Build history of the part. All positions in model axes, mm. A direction names the side the tool comes from. Round coordinates to 2 decimals unless told otherwise and drop trailing zeros. Order: outer loops, then holes, each group sorted by start corner. A loop starts at its lowest first (then second) coordinate and runs counter-clockwise, first axis right, second up. Notation, with made-up numbers: (51.25, 26) -> (63.25, 26) arc R17 ccw to (63.25, 50) -> close; hole circle Ø5 at (-33.5, 16). An arc over 180 degrees is marked (long way). Answer as a JSON object with one key per item and string values.
from build123d import *

# Parameters (mm, degrees)
SKETCH1_R                = 18
SKETCH1_R_2              = 17.75
BOSS_EXTRUDE1_DEPTH      = 210
BOSS_EXTRUDE2_DEPTH      = 22.5
CUT_EXTRUDE2_DEPTH       = 213.245370912
CUT_EXTRUDE12_START      = -27
CUT_EXTRUDE12_DEPTH      = 23.323952
CUT_EXTRUDE13_REACH      = 217.691
CUT_EXTRUDE13_END_RADIUS = 19.770854308
BOSS_EXTRUDE3_REACH      = 235.245
BOSS_EXTRUDE3_END_RADIUS = 18
BOSS_EXTRUDE3_START      = 21


with BuildPart() as part:
    # Sketch1 → Boss-Extrude1 (new body)
    with BuildSketch(Plane(origin=(0, 0, 0), x_dir=(0, 0, -1), z_dir=(1, 0, 0))):
        Circle(SKETCH1_R)
        Circle(SKETCH1_R_2, mode=Mode.SUBTRACT)
    extrude(amount=BOSS_EXTRUDE1_DEPTH)


with BuildPart() as body_2:
    # Sketch4 → Boss-Extrude2 (new, symmetric)
    with BuildSketch(Plane.ZY.offset(-67)):
        with BuildLine():
            ThreePointArc((-13.779943134, 14.177441493), (7.695629669, 18.21164364), (19.770854308, 0))
            add(Edge.make_bspline(
                [(-13.779943134, 14.177441493), (-10.685751008, 18.612681967), (-3.179720318, 24.881089629), (14.245409909, 21.177624873), (20.93871501, 8.550633365), (19.770854308, 0)],
                knots=[0, 0, 0, 0, 0.331280275, 0.485623577, 1, 1, 1, 1], degree=3))
        make_face()
    extrude(amount=BOSS_EXTRUDE2_DEPTH, both=True)


with BuildPart() as cut_extrude2_tool:
    # Sketch2 → Cut-Extrude2 (new, through all)
    with BuildSketch(Plane(origin=(0, 0, 0), x_dir=(1, 0, 0), z_dir=(0, 1, 0))):
        with BuildLine():
            Line((63, -5), (71, -5))
            ThreePointArc((71, -5), (76, 0), (71, 5))
            Line((71, 5), (63, 5))
            ThreePointArc((63, 5), (58, 0), (63, -5))
        make_face()
    extrude(amount=CUT_EXTRUDE2_DEPTH)


with BuildPart() as part_1:
    add(part.part)

    # Cut-Extrude2: cut by cut_extrude2_tool
    add(cut_extrude2_tool.part, mode=Mode.SUBTRACT)



with BuildPart() as body_2_1:
    add(body_2.part)

    # Cut-Extrude2: cut by cut_extrude2_tool
    add(cut_extrude2_tool.part, mode=Mode.SUBTRACT)

    # Sketch7 → Cut-Extrude12 (cut)
    with BuildSketch(Plane(origin=(0, 27, 0), x_dir=(1, 0, 0), z_dir=(0, 1, 0)).offset(CUT_EXTRUDE12_START)):
        with BuildLine():
            ThreePointArc((46.185450517, -14.355615707), (44.923728597, -8.827176662), (44.5, -3.172441075))
            Line((44.5, -3.172441075), (44.5, -19.93558029))
            Line((44.5, -19.93558029), (67, -19.93558029))
            ThreePointArc((67, -19.93558029), (56.225243913, -18.516387819), (46.185450517, -14.355615707))
        make_face()
        with BuildLine():
            ThreePointArc((87.814549483, -14.355615707), (77.774756087, -18.516387819), (67, -19.93558029))
            Line((67, -19.93558029), (89.5, -19.93558029))
            Line((89.5, -19.93558029), (89.5, -3.172440538))
            ThreePointArc((89.5, -3.172440538), (89.076271443, -8.827176396), (87.814549483, -14.355615707))
        make_face()
    extrude(amount=CUT_EXTRUDE12_DEPTH, mode=Mode.SUBTRACT)

    # Cut-Extrude13: up to this cylinder (the profile starts outside it)
    cut_extrude13_end = Plane(origin=(67, 0, 0), z_dir=(1, 0, 0)) * Cylinder(CUT_EXTRUDE13_END_RADIUS, 512.063876616, mode=Mode.PRIVATE)
    # Sketch7<4> → Cut-Extrude13 (cut, up to the surface)
    with BuildSketch(Plane(origin=(0, 27, 0), x_dir=(1, 0, 0), z_dir=(0, 1, 0)), mode=Mode.PRIVATE) as cut_extrude13_sk1:
        with BuildLine():
            Line((62.018448737, 13.779943134), (44.5, 13.779943134))
            Line((44.5, 13.779943134), (44.5, -3.172441075))
            ThreePointArc((44.5, -3.172441075), (44.781644245, 1.442087549), (45.622395888, 5.98811159))
            ThreePointArc((45.622395888, 5.98811159), (53.132553103, 11.331484209), (62.018448737, 13.779943134))
        make_face()
    cut_extrude13_tool1 = extrude(cut_extrude13_sk1.sketch, amount=-CUT_EXTRUDE13_REACH, mode=Mode.PRIVATE) - cut_extrude13_end
    add(cut_extrude13_tool1.solids().sort_by_distance((48.929916, 27, -10.778916))[0], mode=Mode.SUBTRACT)
    # Sketch7<4> → Cut-Extrude13 (cut, up to the surface)
    with BuildSketch(Plane(origin=(0, 27, 0), x_dir=(1, 0, 0), z_dir=(0, 1, 0)), mode=Mode.PRIVATE) as cut_extrude13_sk2:
        with BuildLine():
            Line((89.5, 13.779943134), (71.981551263, 13.779943134))
            ThreePointArc((71.981551263, 13.779943134), (80.867446897, 11.331484209), (88.377604112, 5.98811159))
            ThreePointArc((88.377604112, 5.98811159), (89.218355722, 1.442087815), (89.5, -3.172440538))
            Line((89.5, -3.172440538), (89.5, 13.779943134))
        make_face()
    cut_extrude13_tool2 = extrude(cut_extrude13_sk2.sketch, amount=-CUT_EXTRUDE13_REACH, mode=Mode.PRIVATE) - cut_extrude13_end
    add(cut_extrude13_tool2.solids().sort_by_distance((85.070084, 27, -10.778916))[0], mode=Mode.SUBTRACT)


with BuildPart() as part_2:
    add(part_1.part)

    add(body_2_1.part)  # Boss-Extrude3 merges body 2
    # Boss-Extrude3: up to this cylinder (the profile starts outside it)
    boss_extrude3_end = Plane(origin=(67, 0, 0), z_dir=(-1, 0, 0)) * Cylinder(BOSS_EXTRUDE3_END_RADIUS, 507.49, mode=Mode.PRIVATE)
    # Sketch2<3> → Boss-Extrude3 (add, up to the surface)
    with BuildSketch(Plane(origin=(0, 0, 0), x_dir=(1, 0, 0), z_dir=(0, 1, 0)).offset(BOSS_EXTRUDE3_START), mode=Mode.PRIVATE) as boss_extrude3_sk1:
        with BuildLine():
            Line((62.5, -5.5), (71.5, -5.5))
            ThreePointArc((71.5, -5.5), (77, 0), (71.5, 5.5))
            Line((71.5, 5.5), (62.5, 5.5))
            ThreePointArc((62.5, 5.5), (57, 0), (62.5, -5.5))
        make_face()
        with BuildLine():
            ThreePointArc((71, -5), (76, 0), (71, 5))
            Line((71, 5), (63, 5))
            ThreePointArc((63, 5), (58, 0), (63, -5))
            Line((63, -5), (71, -5))
        make_face(mode=Mode.SUBTRACT)
    boss_extrude3_tool1 = extrude(boss_extrude3_sk1.sketch, amount=-BOSS_EXTRUDE3_REACH, mode=Mode.PRIVATE) - boss_extrude3_end
    add(boss_extrude3_tool1.solids().sort_by_distance((67, 21, 5.271746))[0])


solid = part_2.part
1) Flat gauge pins, fed straight in: pin 1 Ø0.9 at (x, y) = (68.5, 18) entering from +Z; pin 2 Ø1.5 at (x, y) = (153.5, 4) entering from -Z; pin 3 Ø5 at (y, z) = (19, -11.5) entering from -X. Where does each tip first touch, or does it go through?
Checked values:
{"pin 1": "stops at z = 13.78", "pin 2": "stops at z = -17.7", "pin 3": "stops at x = 49.16"}
2) Cut at A-A, the plane y = -5.5. Give the cut face in (x, z).
Checked values:
{"outline": "(0, -17.14) -> (210, -17.14) -> (210, -16.88) -> (0, -16.88) -> close; (0, 16.88) -> (210, 16.88) -> (210, 17.14) -> (0, 17.14) -> close"}
3) Cut at C-C, the plane z = 9. Count the separate pieces of the cut face and the enclosed holes in it, plus the area to 3 significant figures.
Checked values:
{"separate pieces": "3", "enclosed holes": "0", "area": "285 mm²"}
4) Pull direction Y, two halves, no side cores. Call faces 6 (the face through (103.53, -17.328, 3.848)), 7 (the face through (67, 19, -5)): pulls with the +Y half, pulls with the -Y half, needs draft (parallel to the pull), parting line crosses it, or undercut.
Checked values:
{"face 6": "undercut", "face 7": "needs draft"}
5) Which spindle directions (+Z, -Z, +X, -X, +Y, -Y) get a long thin tool onto all of the face, cutting with end or side? Do faces 1 (the face through (49.53, 18.36, -9.26)), 2 (the face through (56.27, 8.42, 18.53)), 3 (the face through (77.824, 8.419, 18.503)), 4 (the face through (67, 20, 5)), 5 (the face through (83.826, 18.089, -9.686)). Say none if no direction does.
Checked values:
{"face 1": "-Z, -X, +Y", "face 2": "+Z, -X, +Y", "face 3": "+Z, +X, +Y", "face 4": "+Y", "face 5": "-Z, +X, +Y"}
6) Probe L1, parallel to Y at x = 46, z = -3; L2, parallel to Y at x = 120, z = 0; L3, parallel to Z at x = 89.5, y = -1. List the from-to ranges inside material, lowest first. Write a range as from..to.
Checked values:
{"L1": "y = -17.75..-17.49, 17.49..17.75, 19.54..22.77", "L2": "y = -18..-17.75, 17.75..18", "L3": "z = -17.97..-17.72, 17.72..17.97"}
7) Cut at B-B, the plane x = 122. Give the cut face in (y, z).
Checked values:
{"outline": "circle Ø36 at (0, 0); hole circle Ø35.5 at (0, 0)"}
